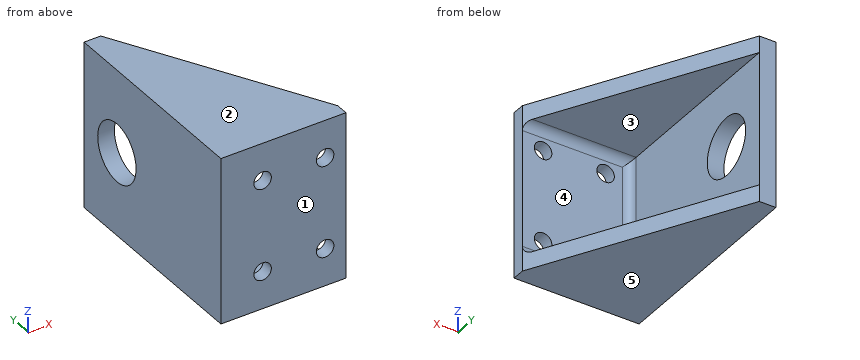
from build123d import *

# Parameters (mm, degrees)
SSS_W               = 30
SSS_H               = 40
SSS_R               = 2.1
BOSS_EXTRUDE2_DEPTH = 3
SKETCH1_W           = 40
SKETCH1_H           = 50
SKETCH1_R           = 7
BOSS_EXTRUDE3_DEPTH = 4
BOSS_EXTRUDE4_DEPTH = 4
FILLET1_R           = 2


with BuildPart() as part:
    # sss → Boss-Extrude2 (new body)
    with BuildSketch(Plane(origin=(0, 0, 0), x_dir=(1, 0, 0), z_dir=(0, 1, 0))):
        with Locations((5, 0)):
            Rectangle(SSS_W, SSS_H)
        with Locations(Location((0, 11, 0), (0, 0, 270))):
            Circle(SSS_R, mode=Mode.SUBTRACT)
        with Locations(Location((0, -11, 0), (0, 0, 90))):
            Circle(SSS_R, mode=Mode.SUBTRACT)
        with Locations(Location((15, -11, 0), (0, 0, 270))):
            Circle(SSS_R, mode=Mode.SUBTRACT)
        with Locations(Location((15, 11, 0), (0, 0, 90))):
            Circle(SSS_R, mode=Mode.SUBTRACT)
    extrude(amount=BOSS_EXTRUDE2_DEPTH)

    # Sketch1 → Boss-Extrude3 (add)
    with BuildSketch(Plane.ZY.offset(10)):
        with Locations((0, 25)):
            Rectangle(SKETCH1_W, SKETCH1_H)
        with Locations((0, 38)):
            Circle(SKETCH1_R, mode=Mode.SUBTRACT)
    extrude(amount=-BOSS_EXTRUDE3_DEPTH)

    # Sketch2 → Boss-Extrude4 (add)
    with BuildSketch(Plane.XY.offset(20)):
        Polygon((-10, 50), (-10, 0), (20, 0), (20, 3), (-6, 50), align=None)
    boss_extrude4 = extrude(amount=-BOSS_EXTRUDE4_DEPTH)

    # Mirror1: Boss-Extrude4 across plane
    add(boss_extrude4.mirror(Plane.XY))

    # Fillet1
    fillet1_edges = [part.edges().sort_by_distance(p)[0] for p in [
        (7, 3, 16),
        (-6, 3, 0),
        (7, 3, -16),
    ]]
    fillet(fillet1_edges, radius=FILLET1_R)


solid = part.part
Could you check a few things on this model? Use its own coordinates, in mm. Face numbers are marked on the shaded views. A direction names the side the tool comes from. Give positions to 0.01 mm unless a question says otherwise; leave off trailing zeros. Order: outer loops, then holes, each group sorted by start corner. A loop starts at its lowest first (then second) coordinate and runs counter-clockwise, first axis right, second up.
Item 1: I need wall thicknesses on line 1 (X direction, y = 1, z = -11); line 2 (Z direction, x = -4.5, y = 36.5); line 3 (X direction, y = 12.5, z = 11.5). Which ranges of each line are inside material? Lowest first, please.
Item 2: If we section it at C-C, the plane y = 42: Write out the boundary of the cut face in (x, z).
Item 3: If we mould it in two halves opening along Z, with no side actions, what happens to the marked faces 1, 2 and 3? For each: pulls with the +Z half, pulls with the -Z half, needs draft (parallel to the pull), parting line crosses it, or undercut.
Item 4: I'm going to push flat-ended pins straight in: pin 1 (2 mm diameter, centred on x = 15, z = -14, fed in from +Y); pin 2 (5 mm diameter, centred on y = 35, z = -5, fed in from -X); pin 3 (22.5 mm diameter, centred on y = 38, z = 0, fed in from +X); pin 4 (7 mm diameter, centred on x = 9, z = 4.5, fed in from +Y). Where does each tip first touch, or does it pass through?
Item 5: If we section it at B-B, the plane x = 15: Write out the boundary of the cut face in (y, z).
Item 6: If we section it at A-A, the plane z = -11: Write out the boundary of the cut face in (x, y), plus the area to 3 significant figures.
Item 7: For the marked faces 4 and 5, which set-ups out of +Z, -Z, +X, -X, +Y, -Y let a thin tool reach every point of the face, with its end or its side?
Item 8: If we section it at D-D, the plane z = 4.5: Write out the boundary of the cut face in (x, y), plus the area to 3 significant figures.
Values:
1. line 1: x = -10 to -2.1, 2.1 to 12.9, 17.1 to 20
1. line 2: z = -20 to -16, 16 to 20
1. line 3: x = -10 to -6
2. outline: (-10, -20) - (-1.57, -20) - (-1.57, -16) - (-6, -16) - (-6, -5.74) - (-10, -5.74) - close; (-10, 5.74) - (-6, 5.74) - (-6, 16) - (-1.57, 16) - (-1.57, 20) - (-10, 20) - close
3. face 1: needs draft
3. face 2: pulls with the +Z half
3. face 3: undercut
4. pin 1: stops at y = 3.27
4. pin 2: stops at x = -10
4. pin 3: stops at x = -6
4. pin 4: stops at y = 3
5. outline: (0, -20) - (12.04, -20) - (12.04, -16) - (5, -16) arc R2 cw to (3, -14) - (3, -13.1) - (0, -13.1) - close; (0, -8.9) - (3, -8.9) - (3, 8.9) - (0, 8.9) - close; (0, 13.1) - (3, 13.1) - (3, 14) arc R2 cw to (5, 16) - (12.04, 16) - (12.04, 20) - (0, 20) - close
6. outline: (-10, 0) - (-2.1, 0) - (-2.1, 3) - (-4, 3) arc R2 cw to (-6, 5) - (-6, 50) - (-10, 50) - close; (2.1, 0) - (12.9, 0) - (12.9, 3) - (2.1, 3) - close; (17.1, 0) - (20, 0) - (20, 3) - (17.1, 3) - close
6. area: 254 mm2
7. face 4: +X, +Y
7. face 5: -Z, +X, -X, +Y, -Y
8. outline: (-10, 0) - (20, 0) - (20, 3) - (-4, 3) arc R2 cw to (-6, 5) - (-6, 32.64) - (-10, 32.64) - close; (-10, 43.36) - (-6, 43.36) - (-6, 50) - (-10, 50) - close
8. area: 236 mm2
